CAD build for the part. Positions are in the model's coordinates, mm. Round coordinates to 2 decimals unless told otherwise and drop trailing zeros. Loops run counter-clockwise (first coordinate to the right, second up) from the corner with the lowest first, then second, coordinate; pieces in that order, holes last.
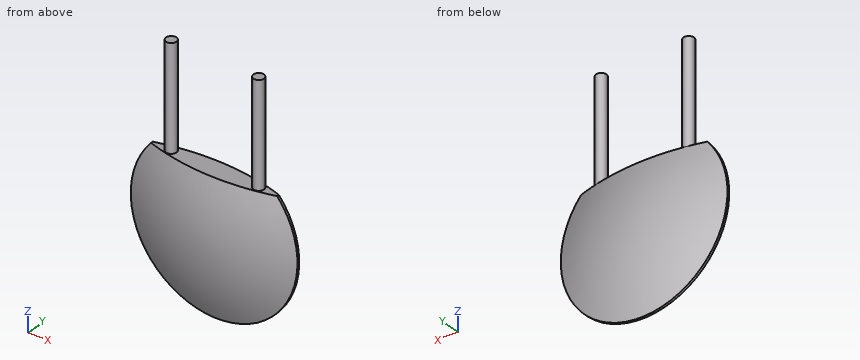
```python
from build123d import *

# Parameters (mm, degrees)
SKETCH_3_W          = 5.794555575
SKETCH_3_H          = 0.933674237
CUT_EXTRUDE_1_DEPTH = 5
SKETCH_4_R          = 0.15
EXTRUDE_1_DEPTH     = 3


with BuildPart() as part:
    # 草图1 → 旋转1 (revolve)
    with BuildSketch(Plane(origin=(0, 0, 0), x_dir=(0, 0, -1), z_dir=(1, 0, 0))):
        with BuildLine():
            Line((0, 0.5), (0, -0.5))
            ThreePointArc((0, -0.5), (1.232422751, -0.38209481), (2.420135029, -0.032656665))
            Line((2.420135029, -0.032656665), (2.420135029, 0.032656665))
            ThreePointArc((2.420135029, 0.032656665), (1.232422751, 0.38209481), (0, 0.5))
        make_face()
    revolve(axis=Axis((0, -1000, 0), (0, 1, 0)))

    # 草图3 → 切除-拉伸1 (cut, symmetric)
    with BuildSketch(Plane(origin=(0, 0, 0), x_dir=(1, 0, 0), z_dir=(0, 1, 0))):
        with Locations((0.081816815, -2.050233119)):
            Rectangle(SKETCH_3_W, SKETCH_3_H)
    extrude(amount=CUT_EXTRUDE_1_DEPTH, both=True, mode=Mode.SUBTRACT)

    # 草图4 → 凸台-拉伸1 (add)
    with BuildSketch(Plane.XY.offset(1.583396)):
        with Locations(Location((-1.27, 0, 0), (0, 0, 180))):
            Circle(SKETCH_4_R)
        with Locations(Location((1.27, 0, 0), (0, 0, 180))):
            Circle(SKETCH_4_R)
    extrude(amount=EXTRUDE_1_DEPTH)


solid = part.part
```
Item 1: Cut at C-C, the plane z = 0. Give the cut face in (x, y).
Answers follow:
outline: (-2.42, -0.03) arc R6.5 ccw to (2.42, -0.03) - (2.42, 0.03) arc R6.5 ccw to (-2.42, 0.03) - close
Item 2: Cut at A-A, the plane z = 2.75. Give the cut face in (x, y), plus the area to 3 significant figures.
Answers follow:
outline: circle Ø0.3 at (-1.27, 0); circle Ø0.3 at (1.27, 0)
area: 0.141 mm2
Item 3: Probe line 1 (Y direction, x = 1.25, z = 4); line 2 (Y direction, x = -1.9, z = 0.5); line 3 (Z direction, x = -2.1, y = 0). List the from-to ranges inside material, lowest first.
Answers follow:
line 1: y = -0.15 to 0.15
line 2: y = -0.2 to 0.2
line 3: z = -1.2 to 1.2
Item 4: Flat gauge pin, fed straight in: P1, Ø2, axis at x = 1, z = -1, coming from the +Y side. Where does the tip first touch, or does it go through?
Answers follow:
P1: stops at y = 0.49
